Check sheet for the modelled part. Datum: model origin and axes. Units: mm. A direction names the side the tool comes from. Give positions to 0.01 mm unless a question says otherwise; leave off trailing zeros. Order: outer loops, then holes, each group sorted by start corner. A loop starts at its lowest first (then second) coordinate and runs counter-clockwise, first axis right, second up. Notation, with made-up numbers: M -24.5,78 L -1.5,78 A33 ccw -1.5,109 Z; hole C 81,34.5 d10. An arc over 180 degrees is marked long. Answer in a Markdown table with one row per item. Add a question column.
from build123d import *

# Parameters (mm, degrees)
CROQUIS1_W              = 180
CROQUIS1_H              = 180
SALIENTE_EXTRUIR1_DEPTH = 30.7
CROQUIS2_W              = 162.21
CROQUIS2_H              = 162.99
CORTAR_EXTRUIR1_DEPTH   = 20.7
CROQUIS4_W              = 175
CROQUIS4_H              = 10.7
CORTAR_EXTRUIR2_DEPTH   = 175
CROQUIS5_W              = 38
CROQUIS5_H              = 40
CORTAR_EXTRUIR3_DEPTH   = 10
CROQUIS6_W              = 38
CROQUIS6_H              = 82.99
CORTAR_EXTRUIR4_DEPTH   = 5
CROQUIS7_W              = 97.21
CROQUIS7_H              = 6.8
CORTAR_EXTRUIR5_DEPTH   = 5
CHAFL_N1_SIZE           = 15
CHAFL_N1_SIZE2          = 8.660254038
CROQUIS8_R              = 1.4
CORTAR_EXTRUIR6_DEPTH   = 20


with BuildPart() as part:
    # Croquis1 → Saliente-Extruir1 (new body)
    with BuildSketch(Plane.XY):
        with Locations((90, 90)):
            Rectangle(CROQUIS1_W, CROQUIS1_H)
    extrude(amount=SALIENTE_EXTRUIR1_DEPTH)

    # Croquis2 → Cortar-Extruir1 (cut)
    with BuildSketch(Plane(origin=(0, 0, 0), x_dir=(-1, 0, 0), z_dir=(0, 0, -1))):
        with Locations((-98.895, 98.505)):
            Rectangle(CROQUIS2_W, CROQUIS2_H)
    extrude(amount=-CORTAR_EXTRUIR1_DEPTH, mode=Mode.SUBTRACT)

    # Croquis4 → Cortar-Extruir2 (cut)
    with BuildSketch(Plane(origin=(0, 180, 0), x_dir=(1, 0, 0), z_dir=(0, 1, 0))):
        with Locations((92.5, -15.35)):
            Rectangle(CROQUIS4_W, CROQUIS4_H)
    extrude(amount=-CORTAR_EXTRUIR2_DEPTH, mode=Mode.SUBTRACT)

    # Croquis5 → Cortar-Extruir3 (cut)
    with BuildSketch(Plane(origin=(0, 0, 20.7), x_dir=(-1, 0, 0), z_dir=(0, 0, -1))):
        with Locations((-161, 160)):
            Rectangle(CROQUIS5_W, CROQUIS5_H)
        with Locations((-161, 37.01)):
            Rectangle(CROQUIS5_W, CROQUIS5_H)
    extrude(amount=-CORTAR_EXTRUIR3_DEPTH, mode=Mode.SUBTRACT)

    # Croquis6 → Cortar-Extruir4 (cut)
    with BuildSketch(Plane.XY.offset(30.7)):
        with Locations((161, 98.505)):
            Rectangle(CROQUIS6_W, CROQUIS6_H)
    extrude(amount=-CORTAR_EXTRUIR4_DEPTH, mode=Mode.SUBTRACT)

    # Croquis7 → Cortar-Extruir5 (cut)
    with BuildSketch(Plane(origin=(0, 0, 20.7), x_dir=(-1, 0, 0), z_dir=(0, 0, -1))):
        with Locations((-66.395, 176.6)):
            Rectangle(CROQUIS7_W, CROQUIS7_H)
    extrude(amount=-CORTAR_EXTRUIR5_DEPTH, mode=Mode.SUBTRACT)

    # Chaflán1
    chafl_n1_edges = [part.edges().sort_by_distance(p)[0] for p in [
        (98.895, 17.01, 0),
        (17.79, 98.505, 0),
    ]]
    chafl_n1_side = [part.faces().sort_by_distance(p)[0] for p in [
        (2.545584412, 90, 0),
    ]]
    chamfer(chafl_n1_edges, length=CHAFL_N1_SIZE, length2=CHAFL_N1_SIZE2, reference=chafl_n1_side[0])

    # Croquis8 → Cortar-Extruir6 (cut)
    with BuildSketch(Plane(origin=(0, 0, 20.7), x_dir=(-1, 0, 0), z_dir=(0, 0, -1))):
        with Locations((-37.79, 176.6)):
            Circle(CROQUIS8_R)
        with Locations((-95, 176.6)):
            Circle(CROQUIS8_R)
        with Locations((-161, 120)):
            Circle(CROQUIS8_R)
        with Locations((-161, 77.01)):
            Circle(CROQUIS8_R)
    extrude(amount=-CORTAR_EXTRUIR6_DEPTH, mode=Mode.SUBTRACT)


solid = part.part
Q1. Cross-section at D-D (y = 46). Record the boundary of the cut face in (x, z).
Q2. Cross-section at A-A (y = 110.5). Record the boundary of the cut face in (x, z).
Q3. Go/stop test with flat-tipped pins: pin 1 (5 mm diameter, centred on x = 57, z = 21.5, fed in from +Y); pin 2 (3.5 mm diameter, centred on x = 37.79, y = 176.6, fed in from -Z); pin 3 (1.5 mm diameter, centred on x = 70, z = 9.5, fed in from +Y). Record where each tip stops, or that it passes through.
Q4. Cross-section at B-B (z = 14). Record the boundary of the cut face in (x, y), and give its area (4 significant figures).
Q5. Tool access check on faces 4 (the flat face through (17.79, 177, 23)), 5 (the flat face through (161, 140, 23)), 6 (the flat face through (10.39, 89.76, 4.39)), 7 (the flat face through (5, 94, 15)), 8 (the flat face through (161, 57.01, 23)). Record the directions out of +Z, -Z, +X, -X, +Y, -Y that give a thin tool (end or side, any length) a straight path to the whole face; none if there is none.
Q6. Thickness scan on probe 1 along Y at (x, z) = (161, 21.7); probe 2 along X at (y, z) = (176.6, 28.2); probe 3 along X at (y, z) = (77.01, 24.5). Record the ranges inside material, lowest first.
Q7. Cross-section at C-C (x = 75). Record the boundary of the cut face in (y, z).
Q8. Draft check along X on faces 1 (the flat face through (180, 98, 23)), 2 (the flat face through (91, 5, 15)), 3 (the flat face through (115, 177, 23)). Enter one of: pulls with the +X half, pulls with the -X half, needs draft (parallel to the pull), parting line crosses it, or undercut.
Values follow:
| question | item | result |
|---|---|---|
| 1 | outline | M 0,0 L 2.79,0 L 17.79,8.66 L 17.79,10 L 5,10 L 5,20.7 L 142,20.7 L 142,30.7 L 0,30.7 Z |
| 2 | outline | M 0,0 L 2.79,0 L 17.79,8.66 L 17.79,10 L 5,10 L 5,20.7 L 180,20.7 L 180,25.7 L 142,25.7 L 142,30.7 L 0,30.7 Z |
| 3 | pin 1 | y = 173.2 |
| 3 | pin 2 | z = 25.7 |
| 3 | pin 3 | y = 17.01 |
| 4 | outline | M 0,0 L 180,0 L 180,5 L 5,5 L 5,180 L 0,180 Z |
| 4 | area | 1,775 mm² |
| 5 | face 4 | -Z, +Y |
| 5 | face 5 | +Z, -Z, +X, +Y |
| 5 | face 6 | -Z, +X, +Y |
| 5 | face 7 | +X, +Y |
| 5 | face 8 | +Z, -Z, +X |
| 6 | probe 1 | 0 to 17.01, 57.01 to 75.61, 78.41 to 118.6, 121.4 to 140 |
| 6 | probe 2 | 0 to 36.39, 39.19 to 93.6, 96.4 to 142 |
| 6 | probe 3 | 0 to 159.6, 162.4 to 180 |
| 7 | outline | M 0,0 L 2.01,0 L 17.01,8.66 L 17.01,10 L 5,10 L 5,20.7 L 173.2,20.7 L 173.2,25.7 L 180,25.7 L 180,30.7 L 0,30.7 Z |
| 8 | face 1 | pulls with the +X half |
| 8 | face 2 | needs draft |
| 8 | face 3 | undercut |
